Model file for the job. Use its own axes, mm. A direction names the side the tool comes from. Coordinates: 2 decimals unless noted, no trailing zeros. Write each loop counter-clockwise with the first axis right and the second up, starting at its lowest first coordinate (ties: lowest second). Pieces come first, ordered by that corner, then holes. Notation, with made-up numbers: M 78.5,-2 L 115.5,-2 A12 cw 115.5,5 Z; hole C -29,73 d4. An arc over 180 degrees is marked long. One line per question, with ' | ' between items. Start each with the question number.
(1) Flat gauge pins, fed straight in: pin 1 Ø5.5 at (x, z) = (13.5, 18.5) entering from -Y; pin 2 Ø10 at (y, z) = (-4.5, -12.5) entering from +X; pin 3 Ø1.5 at (x, z) = (-37.5, -6) entering from +Y. Where does each tip first touch, or does it go through?
(2) Tool access for faces 5 (the face through (0, -20, 18)), 6 (the face through (-12, -12.5, -17)), 7 (the face through (27.854, -7.605, -8.176)), 8 (the face through (-7.5, -16, 18)): list every direction of +Z, -Z, +X, -X, +Y, -Y with a clear straight run to the whole face (end or side of a thin tool).
(3) Two-plate mould, pull along Z, no slides. Class faces 1 (the face through (-31.425, -7.605, 5.603)), 2 (the face through (-0.08, -16.12, -14.62)), 3 (the face through (0, -10, 20)), 4 (the face through (-26.241, -8.935, -17.465)): +Z half, -Z half, draft (parallel to the pull), parting line (faces both ways), or undercut.
(4) Wall check: probe 1 along Z at (x, y) = (30, -9.25); probe 2 along X at (y, z) = (-15.25, 7); probe 3 along Z at (x, y) = (36, -14.5). Give the ranges that are in metal, low to high.
(5) Cut at C-C (y = -18.75). Write the cut outline in (x, z), plus the area to 3 significant figures.
(6) Cut at A-A (y = -8.5). Write the cut outline in (x, z).
(7) Cut at B-B (z = 10.5). Write the cut outline in (x, y), plus the area to 3 significant figures.
from build123d import *

# Parameters (mm, degrees)
BOSS_EXTRUDE1_DEPTH       = 20
BOSS_EXTRUDE2_DEPTH       = 15
F_3_0MM_DOWEL_HOLE1_D     = 4.5
F_3_0MM_DOWEL_HOLE1_DEPTH = 15
F_3_0MM_DOWEL_HOLE1_TIP   = 1.351936393


with BuildPart() as part:
    # Sketch1 → Boss-Extrude1 (new, symmetric)
    with BuildSketch(Plane.XY):
        with BuildLine():
            Line((-30, 0), (-25, 0))
            ThreePointArc((-25, 0), (-17.5, -7.5), (-10, 0))
            Line((-10, 0), (10, 0))
            ThreePointArc((10, 0), (17.5, -7.5), (25, 0))
            Line((25, 0), (30, 0))
            ThreePointArc((30, 0), (26.338834765, -8.838834765), (17.5, -12.5))
            Line((17.5, -12.5), (7.5, -12.5))
            Line((7.5, -12.5), (7.5, -20))
            Line((7.5, -20), (-7.5, -20))
            Line((-7.5, -20), (-7.5, -12.5))
            Line((-7.5, -12.5), (-17.5, -12.5))
            ThreePointArc((-17.5, -12.5), (-26.338834765, -8.838834765), (-30, 0))
        make_face()
    extrude(amount=BOSS_EXTRUDE1_DEPTH, both=True)

    # Sketch6 → Boss-Extrude2 (add, symmetric)
    with BuildSketch(Plane.XY):
        with BuildLine():
            Line((-35, 0), (-35, -10))
            Line((-35, -10), (-40.106769961, -10))
            Line((-40.106769961, -10), (-40.106769961, -25))
            Line((-40.106769961, -25), (-17.606769961, -25))
            Line((-17.606769961, -25), (-22.606769961, -20.683563485))
            Line((-22.606769961, -20.683563485), (22.606769961, -20.683563485))
            Line((22.606769961, -20.683563485), (17.606769961, -25))
            Line((17.606769961, -25), (40.106769961, -25))
            Line((40.106769961, -25), (40.106769961, -10))
            Line((40.106769961, -10), (35, -10))
            Line((35, -10), (35, 0))
            Line((35, 0), (30, 0))
            ThreePointArc((30, 0), (26.338834765, -8.838834765), (17.5, -12.5))
            Line((17.5, -12.5), (7.5, -12.5))
            Line((7.5, -12.5), (7.5, -20))
            Line((7.5, -20), (-7.5, -20))
            Line((-7.5, -20), (-7.5, -12.5))
            Line((-7.5, -12.5), (-17.5, -12.5))
            ThreePointArc((-17.5, -12.5), (-26.338834765, -8.838834765), (-30, 0))
            Line((-30, 0), (-35, 0))
        make_face()
    extrude(amount=BOSS_EXTRUDE2_DEPTH, both=True)

    # Ø3.0mm Dowel Hole1
    with Locations(Plane(origin=(0, 0, 0), x_dir=(1, 0, 0), z_dir=(0, 1, 0))):
        with Locations((0, 15), (0, -15), (30, 7.5), (30, -7.5), (-30, 7.5), (-30.215711777, -7.5)):
            Hole(F_3_0MM_DOWEL_HOLE1_D / 2, depth=F_3_0MM_DOWEL_HOLE1_DEPTH)
            with Locations((0, 0, -(F_3_0MM_DOWEL_HOLE1_DEPTH + F_3_0MM_DOWEL_HOLE1_TIP / 2))):  # 118° drill point
                Cone(0, F_3_0MM_DOWEL_HOLE1_D / 2, F_3_0MM_DOWEL_HOLE1_TIP, mode=Mode.SUBTRACT)


solid = part.part
Filled in:
1) pin 1: y = -12.5 | pin 2: x = 35 | pin 3: y = -10
2) face 5: +Z, +X, -X, -Y | face 6: -Z, -X, -Y | face 7: +Y | face 8: +Z, -X, -Y
3) face 1: undercut | face 2: undercut | face 3: +Z half | face 4: draft
4) probe 1: -15 to -9.75, -5.25 to 5.25, 9.75 to 15 | probe 2: -40.11 to -31.98, -28.45 to 28.24, 31.76 to 40.11 | probe 3: -15 to 15
5) outline: M -40.11,-15 L -7.5,-15 L -7.5,-20 L 7.5,-20 L 7.5,-15 L 40.11,-15 L 40.11,15 L 7.5,15 L 7.5,20 L -7.5,20 L -7.5,15 L -40.11,15 Z | area: 2,560 mm²
6) outline: M -35,-15 L -26.67,-15 L -26.67,-20 L 26.67,-20 L 26.67,-15 L 35,-15 L 35,15 L 26.67,15 L 26.67,20 L -26.67,20 L -26.67,15 L -35,15 Z; hole C -30.22,7.5 d4.5; hole C -30,-7.5 d4.5; hole C 0,-15 d4.5; hole C 0,15 d4.5; hole C 30,-7.5 d4.5; hole C 30,7.5 d4.5
7) outline: M -40.11,-25 L -17.61,-25 L -22.61,-20.68 L 22.61,-20.68 L 17.61,-25 L 40.11,-25 L 40.11,-10 L 35,-10 L 35,0 L 25,0 A7.5 cw 10,0 L -10,0 A7.5 cw -25,0 L -35,0 L -35,-10 L -40.11,-10 Z | area: 1,550 mm²
